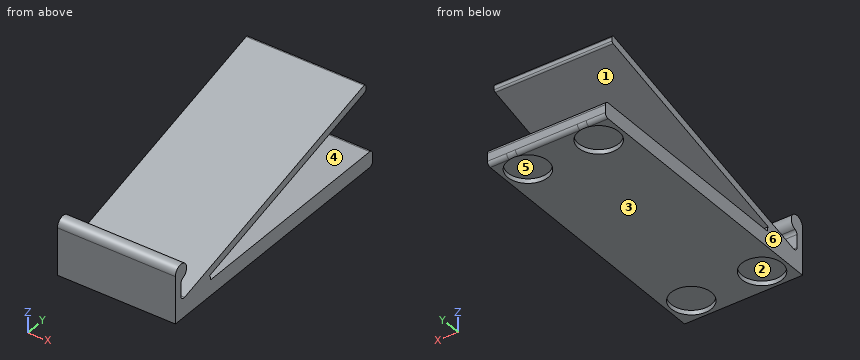
```python
from build123d import *

# Parameters (mm, degrees)
SKETCH_W     = 30
SKETCH_H     = 70
PAD_DEPTH    = 4
PAD001_DEPTH = 30
PAD002_DEPTH = 30
SKETCH003_R  = 5.125
POCKET_DEPTH = 1.15
FILLET_R     = 0.5
FILLET001_R  = 0.5
FILLET002_R  = 1
FILLET003_R  = 1
FILLET004_R  = 1
FILLET005_R  = 1


with BuildPart() as part:
    # Sketch → Pad (new body)
    with BuildSketch(Plane.XY):
        with Locations((15, 35)):
            Rectangle(SKETCH_W, SKETCH_H)
    extrude(amount=PAD_DEPTH)

    # Sketch001 (on Face4 of Pad) → Pad001 (join)
    with BuildSketch(Plane(origin=(0, 0, 0), x_dir=(0, -1, 0), z_dir=(-1, 0, 0))):
        with BuildLine():
            Line((0, 4), (-67.614808, 22.117333))
            Line((-67.614808, 22.117333), (-67.614808, 20.117333))
            Line((-67.614808, 20.117333), (-12.160236, 5.258325))
            ThreePointArc((-12.160236, 5.258325), (-10.651694, 1.586435), (-7.5, 4))
            Line((-7.5, 4), (0, 2))
            Line((0, 2), (0, 4))
        make_face()
    extrude(amount=-PAD001_DEPTH)

    # Sketch002 (on Face5 of Pad001) → Pad002 (join)
    with BuildSketch(Plane(origin=(0, 0, 0), x_dir=(0, -1, 0), z_dir=(-1, 0, 0))):
        with BuildLine():
            Line((0, 0), (-2, 0))
            Line((-2, 0), (-2, 10))
            ThreePointArc((0, 12), (-3.414214, 13.414214), (-2, 10))
            Line((0, 12), (0, 0))
        make_face()
    extrude(amount=-PAD002_DEPTH)

    # Sketch003 (on Face6 of Pad002) → Pocket (cut)
    with BuildSketch(Plane(origin=(0, 0, 0), x_dir=(1, 0, 0), z_dir=(0, 0, -1))):
        with Locations((6, -6)):
            Circle(SKETCH003_R)
        with Locations((24, -6)):
            Circle(SKETCH003_R)
        with Locations((6, -64)):
            Circle(SKETCH003_R)
        with Locations((24, -64)):
            Circle(SKETCH003_R)
    extrude(amount=-POCKET_DEPTH, mode=Mode.SUBTRACT)

    # Fillet
    fillet_edges = [part.edges().sort_by_distance(p)[0] for p in [
        (15, 67.614808, 22.117333),
    ]]
    fillet(fillet_edges, radius=FILLET_R)

    # Fillet001
    fillet001_edges = [part.edges().sort_by_distance(p)[0] for p in [
        (15, 67.614808, 20.117333),
    ]]
    fillet(fillet001_edges, radius=FILLET001_R)

    # Fillet002
    fillet002_edges = [part.edges().sort_by_distance(p)[0] for p in [
        (15, 70, 4),
    ]]
    fillet(fillet002_edges, radius=FILLET002_R)

    # Fillet003
    fillet003_edges = [part.edges().sort_by_distance(p)[0] for p in [
        (15, 70, 0),
    ]]
    fillet(fillet003_edges, radius=FILLET003_R)

    # Fillet004
    fillet004_edges = [part.edges().sort_by_distance(p)[0] for p in [
        (15, 2, 4.535898),
    ]]
    fillet(fillet004_edges, radius=FILLET004_R)

    # Fillet005
    fillet005_edges = [part.edges().sort_by_distance(p)[0] for p in [
        (15, 2, 10),
    ]]
    fillet(fillet005_edges, radius=FILLET005_R)


solid = part.part
```
The model under review builds one solid part; all positions refer to its coordinate system, in mm. Face numbers are marked on the shaded views. A direction names the side the tool comes from. Round coordinates to 2 decimals unless told otherwise and drop trailing zeros. Loops run counter-clockwise (first coordinate to the right, second up) from the corner with the lowest first, then second, coordinate; pieces in that order, holes last. Notation, with made-up numbers: (14, -35.75) - (52, -35.75) arc R29 cw to (52, -15.75) - close; hole circle Ø3 at (38, -1.5). An arc over 180 degrees is marked (long way). Use a Markdown table: item, result. Add a question column.
Q1. The part is to be moulded in two halves that separate along Z. For the marked faces 4, 5 and 6, say which applies: pulls with the +Z half, pulls with the -Z half, needs draft (parallel to the pull), parting line crosses it, or undercut.
Q2. For probe 1 along X at (y, z) = (6, 0.35) (3 decimals); probe 2 along Y at (x, z) = (6, 0.35) (3 decimals); probe 3 along Y at (x, z) = (6, 0.6) (3 decimals), list the stretches that pass through material, from the lowest coordinate up.
Q3. Insertion check: pin 1 Ø1.5 at (y, z) = (25.5, 5.5) entering from -X; pin 2 Ø0.5 at (x, z) = (8, 21) entering from +Y; pin 3 Ø15 at (x, y) = (16.5, 53) entering from +Z; pin 4 Ø8 at (x, y) = (24.5, 5.5) entering from -Z. Each pin has a flat end and moves straight along its axis. Give the tip position at first contact, or say it passes through.
Q4. Add section B-B (y = 64). State the section outline as (x, z) points (3 decimals), plus the area to 3 significant figures.
Q5. Add section C-C (z = 7). State the section outline as (x, y) points.
Q6. Machinability: for the marked faces 1, 2 and 3, which of the approach directions +Z, -Z, +X, -X, +Y, -Y give a long, thin tool a straight path to every point of the face, cutting with its end or side? Answer none if there is none.
Q7. Add section D-D (y = 6). State the section outline as (x, z) points (3 decimals).
Q8. Add section A-A (x = 12). State the section outline as (y, z) points, plus the area to 3 significant figures.
Worked answers:
| question | item | result |
|---|---|---|
| 1 | face 4 | undercut |
| 1 | face 5 | pulls with the -Z half |
| 1 | face 6 | needs draft |
| 2 | probe 1 | 0 to 0.875, 11.125 to 18.875, 29.125 to 30 |
| 2 | probe 2 | 0 to 0.875, 11.125 to 58.875, 69.125 to 69.767 |
| 2 | probe 3 | 0 to 0.875, 11.125 to 58.875, 69.125 to 69.92 |
| 3 | pin 1 | through |
| 3 | pin 2 | y = 67.61 |
| 3 | pin 3 | z = 20.21 |
| 3 | pin 4 | z = 1.15 |
| 4 | outline | (0, 0) - (0.875, 0) - (0.875, 1.15) - (11.125, 1.15) - (11.125, 0) - (18.875, 0) - (18.875, 1.15) - (29.125, 1.15) - (29.125, 0) - (30, 0) - (30, 4) - (0, 4) - close; (0, 19.149) - (30, 19.149) - (30, 21.149) - (0, 21.149) - close |
| 4 | area | 156 mm² |
| 5 | outline | (0, 0) - (30, 0) - (30, 2) - (0, 2) - close; (0, 11.2) - (30, 11.2) - (30, 18.66) - (0, 18.66) - close |
| 6 | face 1 | +X, -X, +Y |
| 6 | face 2 | -Z |
| 6 | face 3 | -Z, +X, -X, +Y, -Y |
| 7 | outline | (0, 0) - (0.875, 0) - (0.875, 1.15) - (11.125, 1.15) - (11.125, 0) - (18.875, 0) - (18.875, 1.15) - (29.125, 1.15) - (29.125, 0) - (30, 0) - (30, 5.608) - (0, 5.608) - close |
| 8 | outline | (0, 0) - (69, 0) arc R1 ccw to (70, 1) - (70, 3) arc R1 ccw to (69, 4) - (12.5, 4) arc R2.5 ccw to (12.16, 5.26) - (67.24, 20.02) arc R0.5 ccw to (67.61, 20.5) - (67.61, 21.47) arc R0.5 ccw to (66.99, 21.95) - (3.26, 4.87) arc R1 cw to (2, 5.84) - (2, 9.17) arc R1 cw to (2.67, 10.11) arc R2 ccw (long way) to (0, 12) - close |
| 8 | area | 436 mm² |
